Verification items for the finished model (mm, model axes). Round coordinates to 2 decimals unless told otherwise and drop trailing zeros. Order: outer loops, then holes, each group sorted by start corner. A loop starts at its lowest first (then second) coordinate and runs counter-clockwise, first axis right, second up. Notation, with made-up numbers: (13, 31.5) -> (59, 31.5) arc R22 cw to (59, 38.5) -> close; hole circle Ø8 at (19.5, 7.25). An arc over 180 degrees is marked (long way). Return JSON: item names as keys, results as strings. Group by question number.
1) Depth check by flat-ended pin: pin 1 (1 mm diameter, centred on y = 2.5, z = 0.5, fed in from -X); pin 2 (0.6 mm diameter, centred on x = -1, z = 0.5, fed in from -Y). Enter the tip coordinate at first touch or a pass-through.
2) Section check A-A on x = -22. Enter the section's corners in (y, z), plus the area to 3 significant figures.
3) Section check C-C on z = 1.4. Enter the section's corners in (x, y).
4) Section check D-D on x = -5.5. Enter the section's corners in (y, z).
5) Section check B-B on y = -2.5. Enter the section's corners in (x, z).
6) Scan lines: L1, parallel to X at y = 0.5, z = 0.3; L2, parallel to X at y = -2.5, z = 0.65; L3, parallel to X at y = 0, z = 1.7. Record each from-to range of solid material in increasing order.
```python
from build123d import *

# Parameters (mm, degrees)
BOSS_EXTRUDE1_DEPTH   = 36.9
M2X0_4_TAPPED_HOLE1_D = 1.6
SKETCH4_W             = 15
SKETCH4_H             = 4.7
CUT_EXTRUDE4_DEPTH    = 38.092452062
FILLET3_R             = 2.5


with BuildPart() as part:
    # Sketch1 → Boss-Extrude1 (new, symmetric)
    with BuildSketch(Plane(origin=(0, 0, 0), x_dir=(0, 0, -1), z_dir=(1, 0, 0))):
        Polygon((0, -3.2), (-2, -1.2), (-2, 3.2), (0, 3.2), align=None)
    extrude(amount=BOSS_EXTRUDE1_DEPTH, both=True)

    # M2x0.4 Tapped Hole1 (through all)
    with Locations(Plane.XY.offset(2)):
        with Locations((22, -0.2), (0, -0.2), (-22, -0.2)):
            Hole(M2X0_4_TAPPED_HOLE1_D / 2)

    # Sketch4 → Cut-Extrude4 (cut, through all)
    with BuildSketch(Plane.XY):
        with Locations((0, -0.85)):
            Rectangle(SKETCH4_W, SKETCH4_H)
    extrude(amount=CUT_EXTRUDE4_DEPTH, mode=Mode.SUBTRACT)

    # Fillet3
    fillet3_edges = [part.edges().sort_by_distance(p)[0] for p in [
        (-36.9, 3.2, 1),
        (36.9, 3.2, 1),
    ]]
    fillet(fillet3_edges, radius=FILLET3_R)


solid = part.part
```
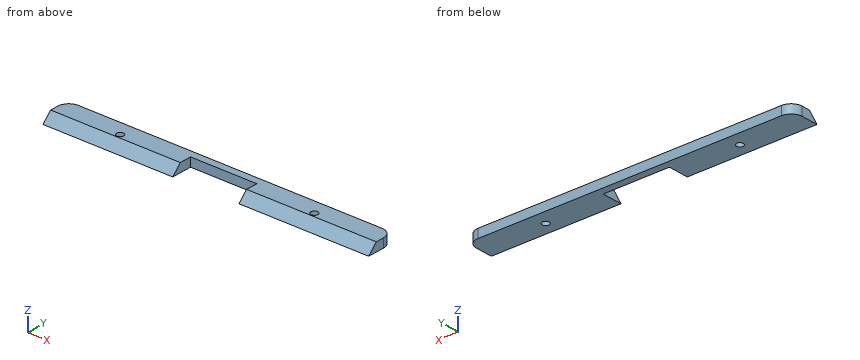
Check result:
{
 "1": {"pin 1": "x = -36.54", "pin 2": "y = 1.5"},
 "2": {"outline": "(-3.2, 0) -> (-1, 0) -> (-1, 2) -> (-1.2, 2) -> close; (0.6, 0) -> (3.2, 0) -> (3.2, 2) -> (0.6, 2) -> close", "area": "7.60 mm^2"},
 "3": {"outline": "(-36.9, -1.8) -> (-7.5, -1.8) -> (-7.5, 1.5) -> (7.5, 1.5) -> (7.5, -1.8) -> (36.9, -1.8) -> (36.9, 0.7) arc R2.5 ccw to (34.4, 3.2) -> (-34.4, 3.2) arc R2.5 ccw to (-36.9, 0.7) -> close; hole circle Ø1.6 at (-22, -0.2); hole circle Ø1.6 at (22, -0.2)"},
 "4": {"outline": "(1.5, 0) -> (3.2, 0) -> (3.2, 2) -> (1.5, 2) -> close"},
 "5": {"outline": "(-36.9, 0) -> (-7.5, 0) -> (-7.5, 0.7) -> (-36.9, 0.7) -> close; (7.5, 0) -> (36.9, 0) -> (36.9, 0.7) -> (7.5, 0.7) -> close"},
 "6": {"L1": "-36.9 to -22.39, -21.61 to -7.5, 7.5 to 21.61, 22.39 to 36.9", "L2": "-36.9 to -7.5, 7.5 to 36.9", "L3": "-36.9 to -22.77, -21.23 to -7.5, 7.5 to 21.23, 22.77 to 36.9"}
}
